Model file for the job. Use its own axes, mm. Face numbers are marked on the shaded views. A direction names the side the tool comes from. Give positions to 0.01 mm unless a question says otherwise; leave off trailing zeros. Order: outer loops, then holes, each group sorted by start corner. A loop starts at its lowest first (then second) coordinate and runs counter-clockwise, first axis right, second up. Notation, with made-up numbers: (35.5, 53) -> (63.5, 53) arc R28 cw to (63.5, 73) -> close; hole circle Ø8 at (48.5, 67.25). An arc over 180 degrees is marked (long way). Use CSV: the item, a comma, the result in double quotes. Start each with the question number.
1. Cut at C-C on z = 18.35. List the corners of the cut face in (x, y).
2. Wall check: line 1 (X direction, y = -3.5, z = 18.35); line 2 (X direction, y = -6.5, z = 36.5); line 3 (Y direction, x = 14.5, z = -21). Give the ranges that are in metal, low to high. Write a range as from..to.
3. 3-axis set-ups, long thin cutter, end or side, ignore diameter. For the marked faces 4 and 5: which of +Z, -Z, +X, -X, +Y, -Y reach the whole face in a straight line?
4. Cut at D-D on x = -32.5. List the corners of the cut face in (y, z) (3 decimals).
5. Cut at A-A on z = 35. List the corners of the cut face in (x, y).
6. Drop flat-ended pins along their axis: pin 1 (11 mm diameter, centred on x = 0, z = 18.35, fed in from +Y); pin 2 (4.5 mm diameter, centred on x = -4, y = -4, fed in from +Z); pin 3 (2 mm diameter, centred on y = -5.5, z = -22, fed in from +X); pin 4 (6 mm diameter, centred on x = -31.5, z = -22, fed in from +Y). Give the stop position or say it passes through.
7. Pull direction X, two halves, no side cores. Call the marked faces 1, 2 and 3: released by +X, released by -X, zero draft, split by the parting line, or undercut.
```python
from build123d import *

# Parameters (mm, degrees)
F1_DEPTH = 9.35
F3_DEPTH = 80.001
F5_DEPTH = 9.351
F6_D     = 9.525


with BuildPart() as f1:
    # F0 (on Front) → F1 (new body)
    with BuildSketch(Plane.XZ):
        with BuildLine():
            Line((-40, -31.95), (40, -31.95))
            Line((40, -31.95), (40, 31.95))
            Line((40, 31.95), (40, 43.95))
            ThreePointArc((40, 43.95), (39.1213203436, 46.0713203436), (37, 46.95))
            Line((37, 46.95), (35, 46.95))
            Line((35, 46.95), (20.8786796564, 32.8286796564))
            ThreePointArc((20.8786796564, 32.8286796564), (19.90540961, 32.1783614025), (18.7573593129, 31.95))
            Line((18.7573593129, 31.95), (-18.7573593129, 31.95))
            ThreePointArc((-18.7573593129, 31.95), (-19.90540961, 32.1783614025), (-20.8786796564, 32.8286796564))
            Line((-20.8786796564, 32.8286796564), (-35, 46.95))
            Line((-35, 46.95), (-37, 46.95))
            ThreePointArc((-37, 46.95), (-39.1213203436, 46.0713203436), (-40, 43.95))
            Line((-40, 43.95), (-40, 31.95))
            Line((-40, 31.95), (-40, -31.95))
        make_face()
    extrude(amount=F1_DEPTH)

    # F2 (on face) → F3 (cut, through all)
    with BuildSketch(Plane.YZ.offset(40)):
        Polygon((0.6493095733, -12.0794061572), (-4.675, -31.95), (-9.9993095733, -12.0794061572), (-14.2520674504, -12.0794061572), (-14.2520674504, -36.8148345501), (6.057018973, -36.8148345501), (6.057018973, -12.0794061572), align=None)
    extrude(amount=-F3_DEPTH, mode=Mode.SUBTRACT)

    # F4 (on face) → F5 (cut, through all)
    with BuildSketch(Plane.XZ.offset(9.35)):
        Polygon((-39.5772941897, -38.7194621272), (-40, -14.5026624746), (-52.0872474203, -14.5026624746), (-52.0872474203, -38.7194621272), align=None)
        Polygon((48.822511771, -14.5026624746), (40, -14.5026624746), (39.5603374031, -39.6909157795), (48.822511771, -39.6909157795), align=None)
    extrude(amount=-F5_DEPTH, mode=Mode.SUBTRACT)

    # F6 (through all)
    with Locations(Plane(origin=(0, 0, 0), x_dir=(1, 0, 0), z_dir=(0, 1, 0))):
        with Locations((0, -18.35)):
            Hole(F6_D / 2)


solid = f1.part
```
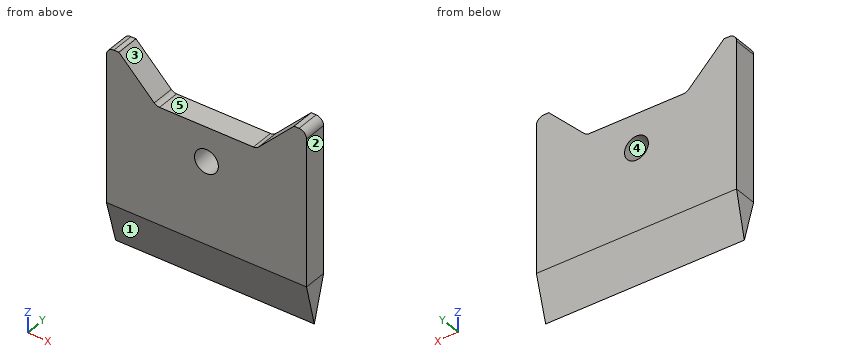
Verdict:
1,outline,"(-40, -9.35) -> (-4.76, -9.35) -> (-4.76, 0) -> (-40, 0) -> close; (4.76, -9.35) -> (40, -9.35) -> (40, 0) -> (4.76, 0) -> close"
2,line 1,"-40..-4.76, 4.76..40"
2,line 2,"-40..-24.55, 24.55..40"
2,line 3,"-7.61..-1.74"
3,face 4,"+Y, -Y"
3,face 5,"+Z, +Y, -Y"
4,outline,"(-9.35, -14.503) -> (-4.675, -31.95) -> (0, -14.503) -> (0, 44.45) -> (-9.35, 44.45) -> close"
5,outline,"(-40, -9.35) -> (-23.05, -9.35) -> (-23.05, 0) -> (-40, 0) -> close; (23.05, -9.35) -> (40, -9.35) -> (40, 0) -> (23.05, 0) -> close"
6,pin 1,"y = 0"
6,pin 2,"z = 31.95"
6,pin 3,"x = 39.89"
6,pin 4,"y = -1.21"
7,face 1,"zero draft"
7,face 2,"released by +X"
7,face 3,"undercut"
